Read the model definition and answer for the solid it produces. Units are mm, in the model's axes. A direction names the side the tool comes from. Coordinates: 2 decimals unless noted, no trailing zeros. Write each loop counter-clockwise with the first axis right and the second up, starting at its lowest first coordinate (ties: lowest second). Pieces come first, ordered by that corner, then holes. Notation, with made-up numbers: (39.25, 2.5) -> (54.25, 2.5) arc R21 cw to (54.25, 35.5) -> close; hole circle Ø10 at (-35, -8). An arc over 180 degrees is marked (long way). One line per item, written item: value. Start each with the question number.
from build123d import *

# Parameters (mm, degrees)
F0_R     = 2.2733
F0_R_2   = 3.991558
F0_R_3   = 11.2522
F1_DEPTH = 7.747


with BuildPart() as f1:
    # F0 (on Top) → F1 (new body)
    with BuildSketch(Plane.XY):
        with BuildLine():
            Line((-10.238358, 36.721247), (-6.219031, 29.75957))
            ThreePointArc((-6.219031, 29.75957), (-7.103307, 19.453476), (-12.983067, 10.943133))
            ThreePointArc((-12.983067, 10.943133), (-13.972901, 0), (-12.983067, -10.943133))
            ThreePointArc((-12.983067, -10.943133), (-7.005384, -19.418275), (-6.219031, -29.75957))
            Line((-6.219031, -29.75957), (-10.238358, -36.721247))
            ThreePointArc((-10.238358, -36.721247), (-10.238358, -39.261247), (-8.038653, -40.531247))
            Line((-8.038653, -40.531247), (8.038653, -40.531247))
            ThreePointArc((8.038653, -40.531247), (10.238358, -39.261247), (10.238358, -36.721247))
            Line((10.238358, -36.721247), (6.219031, -29.75957))
            ThreePointArc((6.219031, -29.75957), (7.103307, -19.453476), (12.983067, -10.943133))
            ThreePointArc((12.983067, -10.943133), (13.972901, 0), (12.983067, 10.943133))
            ThreePointArc((12.983067, 10.943133), (7.005384, 19.418275), (6.219031, 29.75957))
            Line((6.219031, 29.75957), (10.238358, 36.721247))
            ThreePointArc((10.238358, 36.721247), (10.238358, 39.261247), (8.038653, 40.531247))
            Line((8.038653, 40.531247), (-8.038653, 40.531247))
            ThreePointArc((-8.038653, 40.531247), (-10.238358, 39.261247), (-10.238358, 36.721247))
        make_face()
        with Locations((-3.048, -35.44515)):
            Circle(F0_R, mode=Mode.SUBTRACT)
        with Locations((0, -24.129855)):
            Circle(F0_R_2, mode=Mode.SUBTRACT)
        with Locations((3.048, -35.44515)):
            Circle(F0_R, mode=Mode.SUBTRACT)
        Circle(F0_R_3, mode=Mode.SUBTRACT)
        with Locations((0, 24.129855)):
            Circle(F0_R_2, mode=Mode.SUBTRACT)
        with Locations((-3.048, 35.44515)):
            Circle(F0_R, mode=Mode.SUBTRACT)
        with Locations((3.048, 35.44515)):
            Circle(F0_R, mode=Mode.SUBTRACT)
    extrude(amount=F1_DEPTH)


solid = f1.part
1. A cutting plane is placed at C-C on z = 3.5. Give the vertices of the cut face in (x, y), then the cut area to 3 significant figures.
2. For a pull along X with two mould halves and no side action, classify faces 1 (the face through (-7.054, 19.591, 3.819)), 2 (the face through (-3.34, -33.19, 3.82)), 3 (the face through (10.22, -39.29, 3.82)) as +X half, -X half, draft (parallel to the pull), parting line (faces both ways), or undercut.
3. A cutting plane is placed at B-B on x = 0. Give the vertices of the cut face in (y, z), then the cut area to 3 significant figures.
4. A cutting plane is placed at D-D on x = -8.75. Give the vertices of the cut face in (y, z).
5. Given pin 1 (1.5 mm diameter, centred on y = -16.5, z = 3.5, fed in from +X); pin 2 (1.5 mm diameter, centred on x = 10.5, z = 5.5, fed in from -Y); pin 3 (2 mm diameter, centred on x = -10, z = 6, fed in from +Y), each flat-ended and moving along its own axis, determine where each tip first touches the part or whether it passes through.
6. Find the intervals of material crossed by probe 1 along Y at (x, z) = (0, 1.75); probe 2 along X at (y, z) = (34, 3); probe 3 along Y at (x, z) = (-1, 5.5), in increasing order. Write a range as from..to.
7. A tool of negligible diameter and unlimited length cuts with its end or side. For faces 4 (the face through (-3.34, 37.7, 3.82)), 5 (the face through (-8.257, 33.289, 3.819)), 6 (the face through (8.257, -33.289, 3.819)), from which of +Z, -Z, +X, -X, +Y, -Y can it reach the whole face along a straight path? Write none if from no direction.
Derived:
1. outline: (-12.98, -10.94) arc R19.5 cw to (-6.22, -29.76) -> (-10.24, -36.72) arc R2.54 ccw to (-8.04, -40.53) -> (8.04, -40.53) arc R2.54 ccw to (10.24, -36.72) -> (6.22, -29.76) arc R20.16 cw to (12.98, -10.94) arc R60.99 ccw to (12.98, 10.94) arc R19.5 cw to (6.22, 29.76) -> (10.24, 36.72) arc R2.54 ccw to (8.04, 40.53) -> (-8.04, 40.53) arc R2.54 ccw to (-10.24, 36.72) -> (-6.22, 29.76) arc R20.16 cw to (-12.98, 10.94) arc R60.99 ccw to start; hole circle Ø22.5 at (0, 0); hole circle Ø4.55 at (-3.05, -35.45); hole circle Ø4.55 at (-3.05, 35.45); hole circle Ø7.98 at (0, -24.13); hole circle Ø7.98 at (0, 24.13); hole circle Ø4.55 at (3.05, -35.45); hole circle Ø4.55 at (3.05, 35.45)
1. area: 995 mm2
2. face 1: -X half
2. face 2: undercut
2. face 3: +X half
3. outline: (-40.53, 0) -> (-28.12, 0) -> (-28.12, 7.75) -> (-40.53, 7.75) -> close; (-20.14, 0) -> (-11.25, 0) -> (-11.25, 7.75) -> (-20.14, 7.75) -> close; (11.25, 0) -> (20.14, 0) -> (20.14, 7.75) -> (11.25, 7.75) -> close; (28.12, 0) -> (40.53, 0) -> (40.53, 7.75) -> (28.12, 7.75) -> close
3. area: 330 mm2
4. outline: (-40.43, 0) -> (-34.14, 0) -> (-34.14, 7.75) -> (-40.43, 7.75) -> close; (-15.79, 0) -> (-7.07, 0) -> (-7.07, 7.75) -> (-15.79, 7.75) -> close; (7.07, 0) -> (15.96, 0) -> (15.96, 7.75) -> (7.07, 7.75) -> close; (34.14, 0) -> (40.43, 0) -> (40.43, 7.75) -> (34.14, 7.75) -> close
5. pin 1: stops at x = 8.88
5. pin 2: stops at y = -39.87
5. pin 3: stops at y = 40.34
6. probe 1: y = -40.53..-28.12, -20.14..-11.25, 11.25..20.14, 28.12..40.53
6. probe 2: x = -8.67..-4.8, -1.29..1.29, 4.8..8.67
6. probe 3: y = -40.53..-36.43, -34.46..-27.99, -20.27..-11.21, 11.21..20.27, 27.99..34.46, 36.43..40.53
7. face 4: +Z, -Z
7. face 5: +Z, -Z, -X
7. face 6: +Z, -Z, +X
